Geometry: final body of the model. Coordinates: model frame, mm. Face numbers are marked on the shaded views. A direction names the side the tool comes from. Round coordinates to 2 decimals unless told otherwise and drop trailing zeros. Write each loop counter-clockwise with the first axis right and the second up, starting at its lowest first coordinate (ties: lowest second). Pieces come first, ordered by that corner, then holes. Notation, with made-up numbers: (30.5, 71.5) - (89.5, 71.5) arc R17 cw to (89.5, 91.5) - close; hole circle Ø1 at (80.25, 78). An arc over 180 degrees is marked (long way). Write each question's results on one line, items separated by ' | '.
from build123d import *

# Parameters (mm, degrees)
BOSS_EXTRUDE1_DEPTH  = 3.5
SKETCH2_R            = 1.7
CUT_EXTRUDE1_DEPTH   = 14
SKETCH3_R            = 1.7
CUT_EXTRUDE2_DEPTH   = 14
BOSS_EXTRUDE2_DEPTH  = 1
CHAMFER1_SIZE        = 1.5
BOSS_EXTRUDE15_START = -0.9
SKETCH20_R           = 2.9
BOSS_EXTRUDE15_DEPTH = 9.9
FILLET1_R            = 2


with BuildPart() as part:
    # Sketch1 → Boss-Extrude1 (new, symmetric)
    with BuildSketch(Plane(origin=(0, 0, 0), x_dir=(1, 0, 0), z_dir=(0, 1, 0))):
        Polygon((-3.5, 16), (-3.5, -3.5), (16, -3.5), (16, 3.5), (3.5, 3.5), (3.5, 16), align=None)
    extrude(amount=BOSS_EXTRUDE1_DEPTH, both=True)

    # Sketch2 → Cut-Extrude1 (cut)
    with BuildSketch(Plane(origin=(0, 0, -16), x_dir=(-1, 0, 0), z_dir=(0, 0, -1))):
        Circle(SKETCH2_R)
    extrude(amount=-CUT_EXTRUDE1_DEPTH, mode=Mode.SUBTRACT)

    # Sketch3 → Cut-Extrude2 (cut)
    with BuildSketch(Plane(origin=(16, 0, 0), x_dir=(0, 0, -1), z_dir=(1, 0, 0))):
        Circle(SKETCH3_R)
    extrude(amount=-CUT_EXTRUDE2_DEPTH, mode=Mode.SUBTRACT)

    # Sketch4 → Boss-Extrude2 (add, symmetric)
    with BuildSketch(Plane(origin=(0, 0, 0), x_dir=(1, 0, 0), z_dir=(0, 1, 0))):
        Polygon((3.5, 16), (16, 3.5), (3.5, 3.5), align=None)
    extrude(amount=BOSS_EXTRUDE2_DEPTH, both=True)

    # Chamfer1
    chamfer1_edges = [part.edges().sort_by_distance(p)[0] for p in [
        (-3.5, 0, 3.5),
        (6.25, 3.5, 3.5),
        (9.75, 3.5, -3.5),
        (3.5, 3.5, -9.75),
        (3.5, -3.5, -9.75),
        (9.75, -3.5, -3.5),
        (6.25, -3.5, 3.5),
        (-3.5, -3.5, -6.25),
        (-3.5, 3.5, -6.25),
    ]]
    chamfer(chamfer1_edges, length=CHAMFER1_SIZE)

    # Sketch20 → Boss-Extrude15 (add)
    with BuildSketch(Plane.XY.offset(3.5).offset(BOSS_EXTRUDE15_START)):
        with Locations(Location((8.2, 0, 0), (0, 0, 223.602818973))):
            Circle(SKETCH20_R)
    extrude(amount=BOSS_EXTRUDE15_DEPTH)

    # Fillet1
    fillet1_edges = [part.edges().sort_by_distance(p)[0] for p in [
        (10.3, 2, 12.5),
    ]]
    fillet(fillet1_edges, radius=FILLET1_R)


solid = part.part
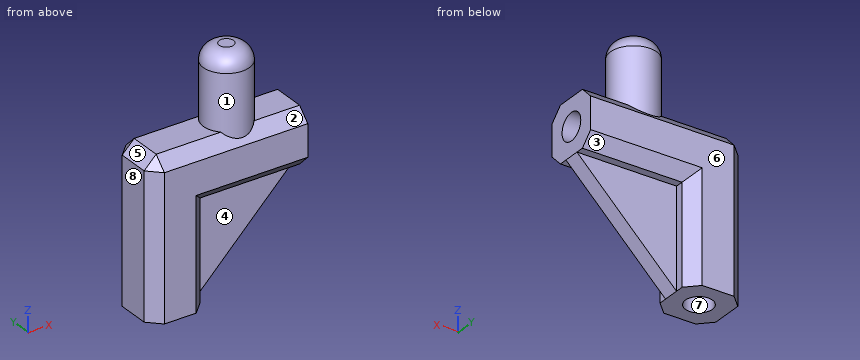
Q1. Ray query, line 1 along Y through (x, z) = (0, -13); line 2 along Y through (x, z) = (11.25, 1.25); line 3 along X through (y, z) = (0.75, -8.5). Return the intervals inside material, ascending.
Answer block:
line 1: -3.5 to -1.7, 1.7 to 3.5 | line 2: -3.5 to -1.15, 1.15 to 3.5 | line 3: -3.5 to -1.53, 1.53 to 11
Q2. Section query C-C, the plane x = 13. Return loops of the section in (y, z), plus the area to 3 significant figures.
Answer block:
outline: (-3.5, -2) - (-2, -3.5) - (-1, -3.5) - (-1, -6.5) - (1, -6.5) - (1, -3.5) - (2, -3.5) - (3.5, -2) - (3.5, 2) - (2, 3.5) - (-2, 3.5) - (-3.5, 2) - close; hole circle Ø3.4 at (0, 0) | area: 41.4 mm2
Q3. Section query B-B, the plane z = -5.5. Return loops of the section in (x, y), plus the area to 3 significant figures.
Answer block:
outline: (-3.5, -2) - (-2, -3.5) - (2, -3.5) - (3.5, -2) - (3.5, -1) - (14, -1) - (14, 1) - (3.5, 1) - (3.5, 2) - (2, 3.5) - (-2, 3.5) - (-3.5, 2) - close; hole circle Ø3.4 at (0, 0) | area: 56.4 mm2
Q4. Pin query (flat end, axial travel): pin 1 (1 mm diameter, centred on y = -0.5, z = 0, fed in from +X); pin 2 (1 mm diameter, centred on x = -1, y = 0, fed in from -Z); pin 3 (4 mm diameter, centred on x = 0, y = 0, fed in from -Z); pin 4 (1.2 mm diameter, centred on x = 14.5, y = -0.5, fed in from +Z). Return the tip coordinate at first contact, or that it passes through.
Answer block:
pin 1: x = 2 | pin 2: z = -2 | pin 3: z = -16 | pin 4: z = 3.5
Q5. Mould query, pull axis Y, two halves, no side actions, for the marked faces 6, 7 and 8. Classes: pulls with the +Y half, pulls with the -Y half, needs draft (parallel to the pull), parting line crosses it, or undercut.
Answer block:
face 6: pulls with the +Y half | face 7: undercut | face 8: needs draft
Q6. Access query for the marked faces 1, 2, 3, 4 and 5. Directions: +Z, -Z, +X, -X, +Y, -Y. A direction counts if a zero-diameter tool reaches every point of the face in a straight line with its end or side. Return the directions, or none.
Answer block:
face 1: +Z | face 2: +Z, -Y | face 3: -Z, +X, +Y | face 4: -Z, +X, -Y | face 5: +Z, -X, +Y, -Y
